For this review, use the dimensioned drawing (mm, ordinates from the lowest corner) and the shaded views. A direction names the side the tool comes from. Give positions to 0.01 mm unless a question says otherwise; leave off trailing zeros. Write each loop counter-clockwise with the first axis right and the second up, starting at its lowest first coordinate (ties: lowest second). Pieces come first, ordered by that corner, then holes.
1) We need section D-D on y = 15. Give the boundary of the cut face in (x, z).
2) We need section C-C on z = 16. Give the boundary of the cut face in (x, y).
3) We need section A-A on x = 4.25. Give the boundary of the cut face in (y, z).
4) Wall thickness on line 1 along Z through (x, y) = (10.25, 93); line 2 along Y through (x, z) = (7, 17.75): over which ranges is each line inside the solid? List them lowest first.
5) Draft analysis for pull direction X (two halves, no side actions). For the marked faces 3, 4 and 5, state which applies: pulls with the +X half, pulls with the -X half, needs draft (parallel to the pull), parting line crosses it, or undercut.
6) Machinability: for the marked faces 1 and 2, which of the approach directions +Z, -Z, +X, -X, +Y, -Y give a long, thin tool a straight path to every point of the face, cutting with its end or side? Answer none if there is none.
7) For P1, Ø8, axis at x = 7.5, y = 74, coming from the -Z side; P2, Ø4, axis at x = 15, z = 9, coming from the +Y side, all flat-tipped, find the tip position at first contact; note any pin that passes through.
8) We need section B-B on y = 37. Give the boundary of the cut face in (x, z).
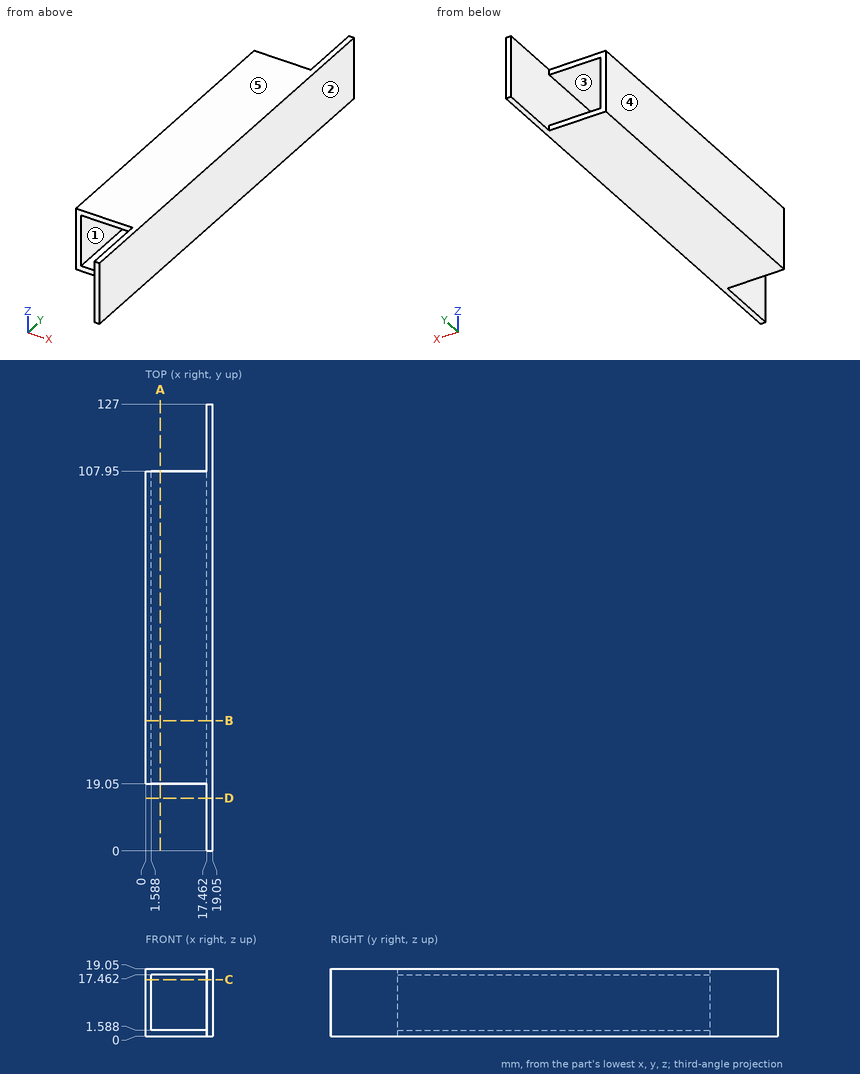
Results list:
1. outline: (17.46, 0) - (19.05, 0) - (19.05, 19.05) - (17.46, 19.05) - close
2. outline: (0, 19.05) - (1.59, 19.05) - (1.59, 107.95) - (0, 107.95) - close; (17.46, 0) - (19.05, 0) - (19.05, 127) - (17.46, 127) - close
3. outline: (19.05, 0) - (107.95, 0) - (107.95, 1.59) - (19.05, 1.59) - close; (19.05, 17.46) - (107.95, 17.46) - (107.95, 19.05) - (19.05, 19.05) - close
4. line 1: z = 0 to 1.59, 17.46 to 19.05
4. line 2: y = 19.05 to 107.95
5. face 3: undercut
5. face 4: pulls with the -X half
5. face 5: needs draft
6. face 1: +Y, -Y
6. face 2: +Z, -Z, +X, +Y, -Y
7. P1: stops at z = 0
7. P2: passes through
8. outline: (0, 0) - (19.05, 0) - (19.05, 19.05) - (0, 19.05) - close; hole (1.59, 1.59) - (17.46, 1.59) - (17.46, 17.46) - (1.59, 17.46) - close
